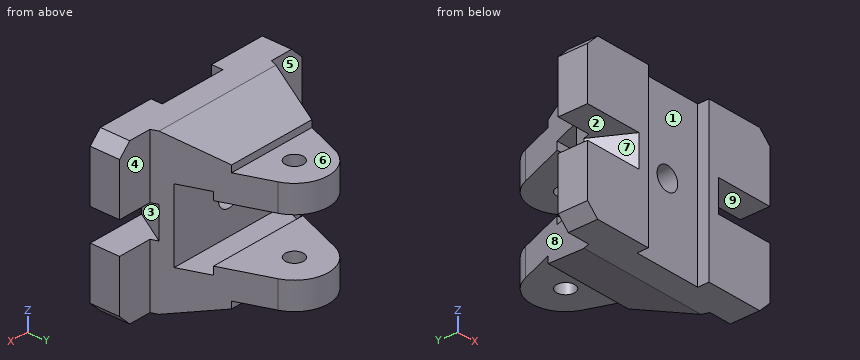
```python
from build123d import *

# Parameters (mm, degrees)
SKETCH1_W                = 70
SKETCH1_H                = 13
BOSS_EXTRUDE1_DEPTH      = 45
CHAMFER1_SIZE            = 5
CUT_EXTRUDE1_DEPTH       = 58.378131723
CUT_EXTRUDE1_DEPTH_BACK  = 58.378131723
SKETCH3_W                = 30
SKETCH3_H                = 5
BOSS_EXTRUDE2_DEPTH      = 35
BOSS_EXTRUDE2_DEPTH_BACK = 35
CUT_EXTRUDE11_DEPTH      = 82.683841731
CUT_EXTRUDE11_DEPTH_BACK = 82.683841731
CUT_EXTRUDE12_DEPTH      = 7
F_8_0_8_DIAMETER_HOLE2_D = 8
M12_TAPPED_HOLE1_D       = 10.2


with BuildPart() as part:
    # Sketch1 → Boss-Extrude1 (new, symmetric)
    with BuildSketch(Plane(origin=(0, 0, 0), x_dir=(0, 0, -1), z_dir=(1, 0, 0))):
        Rectangle(SKETCH1_W, SKETCH1_H)
    extrude(amount=BOSS_EXTRUDE1_DEPTH, both=True)

    # Chamfer1
    chamfer1_edges = [part.edges().sort_by_distance(p)[0] for p in [
        (45, 0, -35),
        (45, 0, 35),
        (-45, 0, -35),
        (-45, 0, 35),
    ]]
    chamfer(chamfer1_edges, length=CHAMFER1_SIZE)

    # Sketch3 → Cut-Extrude1 (cut, two sides: drawn at the far end of the back side and taken through both)
    with BuildSketch(Plane.XY.offset(-CUT_EXTRUDE1_DEPTH_BACK)):
        with Locations((0, -4)):
            Rectangle(SKETCH3_W, SKETCH3_H)
    extrude(amount=CUT_EXTRUDE1_DEPTH + CUT_EXTRUDE1_DEPTH_BACK, mode=Mode.SUBTRACT)

    # Sketch4 → Boss-Extrude2 (add, two sides: drawn at the far end of the back side and taken through both)
    with BuildSketch(Plane.XY.offset(-BOSS_EXTRUDE2_DEPTH_BACK)):
        with BuildLine():
            Line((-30, 6.5), (-14.033447824, 48.797390128))
            ThreePointArc((-14.033447824, 48.797390128), (0, 58.5), (14.033447824, 48.797390128))
            Line((14.033447824, 48.797390128), (30, 6.5))
            Line((30, 6.5), (-30, 6.5))
        make_face()
    extrude(amount=BOSS_EXTRUDE2_DEPTH + BOSS_EXTRUDE2_DEPTH_BACK)

    # Sketch13 → Cut-Extrude11 (cut, two sides: drawn at the far end of the back side and taken through both)
    with BuildSketch(Plane(origin=(0, 0, 0), x_dir=(0, 0, -1), z_dir=(1, 0, 0)).offset(-CUT_EXTRUDE11_DEPTH_BACK)):
        Polygon((-88.955494026, -163.157580884), (-35, 9.5), (-27.5, 33.5), (-24.5, 33.5), (-24.5, 58.5), (-12.5, 58.5), (-12.5, 27.5), (-16, 27.5), (-16, 14.5), (16, 14.5), (16, 27.5), (12.5, 27.5), (12.5, 58.5), (24.5, 58.5), (24.5, 33.5), (27.5, 33.5), (35, 9.5), (88.955494026, -163.157580884), (88.955494026, 198.625976356), (-88.955494026, 198.625976356), align=None)
    extrude(amount=CUT_EXTRUDE11_DEPTH + CUT_EXTRUDE11_DEPTH_BACK, mode=Mode.SUBTRACT)

    # Sketch14 → Cut-Extrude12 (cut, symmetric)
    with BuildSketch(Plane.XY):
        Polygon((28.867550542, 9.5), (19.629946235, -6.5), (45, -6.5), (45, 6.5), (30, 6.5), align=None)
    cut_extrude12 = extrude(amount=CUT_EXTRUDE12_DEPTH, both=True, mode=Mode.SUBTRACT)

    # Mirror1: Cut-Extrude12 across plane
    add(cut_extrude12.mirror(Plane(origin=(0, 0, 0), x_dir=(0, 0, 1), z_dir=(1, 0, 0))), mode=Mode.SUBTRACT)

    # Ø8.0 (8) Diameter Hole2 (through all)
    with Locations(Plane.XY.offset(24.5)):
        with Locations((0, 43.5)):
            Hole(F_8_0_8_DIAMETER_HOLE2_D / 2)

    # M12 Tapped Hole1 (through all)
    with Locations(Plane(origin=(0, 14.5, 0), x_dir=(1, 0, 0), z_dir=(0, 1, 0))):
        with Locations((0, 0)):
            Hole(M12_TAPPED_HOLE1_D / 2)


solid = part.part
```
The listing builds one solid part. Answer for the finished solid, in the listing's coordinates (mm). Face numbers are marked on the shaded views. A direction names the side the tool comes from. Round coordinates to 2 decimals unless told otherwise and drop trailing zeros. Loops run counter-clockwise (first coordinate to the right, second up) from the corner with the lowest first, then second, coordinate; pieces in that order, holes last. Notation, with made-up numbers: (7.25, 3.25) - (34.25, 3.25) arc R34 ccw to (34.25, 34.25) - close; hole circle Ø9 at (77.25, 17.25). An arc over 180 degrees is marked (long way). Use one line per item in the form item = value. Start each with the question number.
1. Given pin 1 Ø9 at (x, z) = (0, 0) entering from +Y; pin 2 Ø2 at (x, y) = (14.5, 27) entering from -Z; pin 3 Ø6.5 at (x, y) = (-10, 22.5) entering from -Z; pin 4 Ø1.5 at (x, z) = (-6.5, 25.5) entering from +Y, each flat-ended and moving along its own axis, determine where each tip first touches the part or whether it passes through.
2. The part is cut by section A-A on z = 0. Determine the outline of the cut face in (x, y).
3. Consider line 1 (Y direction, x = 0, z = 22); line 2 (Y direction, x = 3.5, z = -9); line 3 (Y direction, x = -18, z = 8). Determine where each line is inside the solid, lowest interval first. Write a range as [from, to].
4. The part is cut by section D-D on y = 45. Determine the outline of the cut face in (x, z).
5. A tool of negligible diameter and unlimited length cuts with its end or side. For the marked faces 1, 2, 3, 4 and 5, from which of +Z, -Z, +X, -X, +Y, -Y can it reach the whole face along a straight path? Write none if from no direction.
6. For a pull along Z with two mould halves and no side action, classify the marked faces 6, 7, 8 and 9 as pulls with the +Z half, pulls with the -Z half, needs draft (parallel to the pull), parting line crosses it, or undercut.
7. The part is cut by section C-C on z = 23. Determine the outline of the cut face in (x, y).
8. The part is cut by section B-B on x = 0. Give the number of separate pieces and of enclosed holes in the cut face, then the cut area to 3 significant figures.
Geometry check:
q1.pin_1 = through
q1.pin_2 = -29.84
q1.pin_3 = -31.95
q1.pin_4 = 33.5
q2.outline = (-28.87, 9.5) - (-19.63, -6.5) - (-15, -6.5) - (-15, -1.5) - (-5.1, -1.5) - (-5.1, 14.5) - (-26.98, 14.5) - close; (5.1, -1.5) - (15, -1.5) - (15, -6.5) - (19.63, -6.5) - (28.87, 9.5) - (26.98, 14.5) - (5.1, 14.5) - close
q3.line_1 = [-1.5, 39.5], [47.5, 58.5]
q3.line_2 = [-1.5, 14.5]
q3.line_3 = [-6.5, 14.5]
q4.outline = (-15.47, -24.5) - (-3.71, -24.5) - (-3.71, -12.5) - (-15.47, -12.5) - close; (-15.47, 12.5) - (-3.71, 12.5) - (-3.71, 24.5) - (-15.47, 24.5) - close; (3.71, -24.5) - (15.47, -24.5) - (15.47, -12.5) - (3.71, -12.5) - close; (3.71, 12.5) - (15.47, 12.5) - (15.47, 24.5) - (3.71, 24.5) - close
q5.face_1 = +Z, -Z, -Y
q5.face_2 = -X, -Y
q5.face_3 = +X, -Y
q5.face_4 = +Z, -Z, +X, +Y
q5.face_5 = +Z, -Z, -X, +Y
q6.face_6 = pulls with the +Z half
q6.face_7 = undercut
q6.face_8 = needs draft
q6.face_9 = undercut
q7.outline = (-45, -6.5) - (-15, -6.5) - (-15, -1.5) - (15, -1.5) - (15, -6.5) - (45, -6.5) - (45, 6.5) - (30, 6.5) - (14.03, 48.8) arc R15 ccw to (-14.03, 48.8) - (-30, 6.5) - (-45, 6.5) - close; hole circle Ø8 at (0, 43.5)
q8.separate_pieces = 4
q8.enclosed_holes = 0
q8.area = 1,950 mm^2
